For this review, take the finished solid that the model builds, in its own axes (mm). Face numbers are marked on the shaded views. A direction names the side the tool comes from. Coordinates: 2 decimals unless noted, no trailing zeros. Loops run counter-clockwise (first coordinate to the right, second up) from the corner with the lowest first, then second, coordinate; pieces in that order, holes last. Notation, with made-up numbers: (61, 1) -> (84, 1) arc R15 cw to (84, 9) -> close; hole circle Ø1 at (12.25, 43.5). An arc over 180 degrees is marked (long way). Use a Markdown table: item, result.
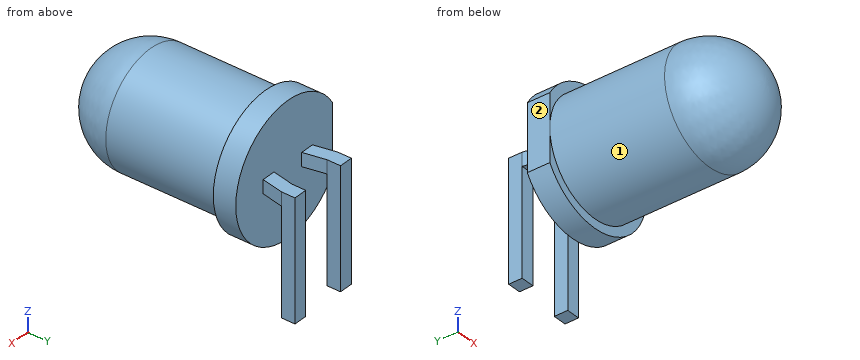
from build123d import *

# Parameters (mm, degrees)
PAD001_DEPTH   = 0.6
SKETCH002_W    = 2.54
SKETCH002_H    = 0.6
PAD002_DEPTH   = 1
SKETCH004_R    = 2.9
SKETCH004_R_2  = 2.5
PAD003_DEPTH   = 1
SKETCH006_W    = 0.4
SKETCH006_H    = 5.8
POCKET_DEPTH   = 1.001
SKETCH_W       = 0.6
SKETCH_H       = 0.6
PAD_DEPTH      = 2.7
PAD_DEPTH_BACK = 2


with BuildPart() as pad001:
    # Sketch001 → Pad001 (new body)
    with BuildSketch(Plane.XY.offset(2.7)):
        Polygon((0.3, 0.3), (-0.3, 0.3), (-0.3, -0.3), (0, -1.77), (0.6, -1.77), (0.3, -0.3), align=None)
        Polygon((2.84, 0.3), (2.24, 0.3), (2.24, -0.3), (1.94, -1.77), (2.54, -1.77), (2.84, -0.3), align=None)
    extrude(amount=PAD001_DEPTH)


with BuildPart() as pad002:
    # Sketch002 → Pad002 (new body)
    with BuildSketch(Plane.XZ.offset(1.77)):
        with Locations((1.27, 3)):
            Rectangle(SKETCH002_W, SKETCH002_H)
    extrude(amount=PAD002_DEPTH)


with BuildPart() as revolution:
    # Sketch003 → Revolution (revolve)
    with BuildSketch(Plane.YZ.offset(1.27)):
        with BuildLine():
            Line((-1.27, 3), (-9.87, 3))
            ThreePointArc((-7.37, 5.5), (-9.137767, 4.767767), (-9.87, 3))
            Line((-1.27, 5.5), (-7.37, 5.5))
            Line((-1.27, 3), (-1.27, 5.5))
        make_face()
    revolve(axis=Axis((1.27, -5.810397, 3), (0, -1, 0)))


with BuildPart() as revolution001:
    # Sketch005 → Revolution001 (revolve)
    with BuildSketch(Plane.YZ.offset(1.27)):
        Polygon((-2.47, 3), (-2.97, 3), (-2.97, 3.5), align=None)
    revolve(axis=Axis((1.27, -3.977201, 3), (0, -1, 0)))


with BuildPart() as pocket:
    # Sketch004 → Pad003 (new body)
    with BuildSketch(Plane.XZ.offset(1.27)):
        with Locations((1.27, 3)):
            Circle(SKETCH004_R)
        with Locations((1.27, 3)):
            Circle(SKETCH004_R_2, mode=Mode.SUBTRACT)
    extrude(amount=PAD003_DEPTH)

    # Sketch006 → Pocket (cut, through all)
    with BuildSketch(Plane.XZ.offset(2.27)):
        with Locations((-1.43, 3)):
            Rectangle(SKETCH006_W, SKETCH006_H)
    extrude(amount=-POCKET_DEPTH, mode=Mode.SUBTRACT)


with BuildPart() as obj1:
    # Sketch → Pad (new body, two sides)
    with BuildSketch(Plane.XY) as pad_sk:
        Rectangle(SKETCH_W, SKETCH_H)
        with Locations((2.54, 0)):
            Rectangle(SKETCH_W, SKETCH_H)
    extrude(amount=PAD_DEPTH)
    extrude(pad_sk.sketch, amount=-PAD_DEPTH_BACK)

    # obj1: union Pad001, Pad002, Revolution, Revolution001, Pocket
    add(pad001.part)
    add(pad002.part)
    add(revolution.part)
    add(revolution001.part)
    add(pocket.part)


solid = obj1.part
(1) Take a section at A-A on z = -1. Write out the cut boundary in (x, y), plus the area to 3 significant figures.
Found:
| item | result |
|---|---|
| outline | (-0.3, -0.3) -> (0.3, -0.3) -> (0.3, 0.3) -> (-0.3, 0.3) -> close; (2.24, -0.3) -> (2.84, -0.3) -> (2.84, 0.3) -> (2.24, 0.3) -> close |
| area | 0.720 mm^2 |
(2) For pin 1 Ø1.5 at (x, y) = (1, -9) entering from +Z; pin 2 Ø0.5 at (y, z) = (0, 0.5) entering from +X; pin 3 Ø3 at (x, y) = (2, -5.5) entering from +Z, all flat-tipped, find the tip position at first contact; note any pin that passes through.
Found:
| item | result |
|---|---|
| pin 1 | stops at z = 5.33 |
| pin 2 | stops at x = 2.84 |
| pin 3 | stops at z = 5.5 |
(3) Take a section at D-D on y = -2. Write out the cut boundary in (x, z), plus the area to 3 significant figures.
Found:
| item | result |
|---|---|
| outline | (-1.23, 1.53) arc R2.9 ccw (long way) to (-1.23, 4.47) -> close |
| area | 25.6 mm^2 |
(4) Take a section at B-B on y = -4. Write out the cut boundary in (x, z).
Found:
| item | result |
|---|---|
| outline | circle Ø5 at (1.27, 3) |
(5) Take a section at C-C on z = 1. State how many separate pieces and enclosed holes the cut face has, plus the area to 3 significant figures.
Found:
| item | result |
|---|---|
| separate pieces | 3 |
| enclosed holes | 0 |
| area | 23.8 mm^2 |
(6) For line 1 along X through (y, z) = (-5.75, 3); line 2 along Y through (x, z) = (-0.65, 1); line 3 along Z through (x, y) = (1.15, -3.75), list the stretches that pass through material, from the lowest coordinate up.
Found:
| item | result |
|---|---|
| line 1 | x = -1.23 to 3.77 |
| line 2 | y = -2.27 to -1.27 |
| line 3 | z = 0.5 to 5.5 |
(7) For the marked faces 1 and 2, list the 3-axis set-ups (+Z, -Z, +X, -X, +Y, -Y) from which the entire face can be reached by the end or side of a thin tool; tool diameter is ignored.
Found:
| item | result |
|---|---|
| face 1 | -Y |
| face 2 | +Z, -Z, -X, +Y, -Y |
